```python
from build123d import *

# Parameters (mm, degrees)
F1_DEPTH      = 85
F2_R          = 2.5
F3_DEPTH      = 45
F4_R          = 2.5
F5_DEPTH      = 15
F5_DEPTH_BACK = 25
F6_R          = 1.5
F7_DEPTH      = 15


with BuildPart() as f1:
    # F0 (on Front) → F1 (new body, symmetric)
    with BuildSketch(Plane.XZ):
        Polygon((42, -15), (45, -15), (45, 15), (-45, 15), (-45, -15), (-42, -15), (-42, 12), (42, 12), align=None)
    extrude(amount=F1_DEPTH, both=True)

    # F2 (on Right) → F3 (join, symmetric)
    with BuildSketch(Plane.YZ):
        with Locations((-75, 0)):
            Circle(F2_R)
        with Locations((75, 0)):
            Circle(F2_R)
    extrude(amount=F3_DEPTH, both=True)

    # F4 (on Top) → F5 (join, two sides)
    with BuildSketch(Plane.XY) as f5_sk:
        with Locations((-30, -50)):
            Circle(F4_R)
        with Locations((30, -50)):
            Circle(F4_R)
        with Locations((30, 50)):
            Circle(F4_R)
        with Locations((-30, 50)):
            Circle(F4_R)
    extrude(amount=F5_DEPTH)
    extrude(f5_sk.sketch, amount=-F5_DEPTH_BACK)

    # F6 (on Top) → F7 (cut)
    with BuildSketch(Plane.XY):
        with Locations((-10, 35)):
            Circle(F6_R)
        with Locations((10, 35)):
            Circle(F6_R)
        with Locations((10, -35)):
            Circle(F6_R)
        with Locations((-10, -35)):
            Circle(F6_R)
        with Locations((-15, 35)):
            Circle(F6_R)
        with Locations((15, 35)):
            Circle(F6_R)
        with Locations((15, -35)):
            Circle(F6_R)
        with Locations((-15, -35)):
            Circle(F6_R)
    extrude(amount=F7_DEPTH, mode=Mode.SUBTRACT)


solid = f1.part
```
Model file for the job. Use its own axes, mm. Coordinates: 2 decimals unless noted, no trailing zeros. Loops run counter-clockwise (first coordinate to the right, second up) from the corner with the lowest first, then second, coordinate; pieces in that order, holes last. Notation, with made-up numbers: (40.25, 51) - (53.25, 51) arc R27 ccw to (53.25, 75) - close; hole circle Ø2 at (-14, 11.25). An arc over 180 degrees is marked (long way). Answer as a JSON object with one key per item and string values. Group by question number.
(1) Probe line 1 along Y through (x, z) = (-10, 14); line 2 along X through (y, z) = (35, 12.9); line 3 along X through (y, z) = (-9, -13.5). List the from-to ranges inside material, lowest first.
(2) Cut at B-B (x = 39). Give the cut face in (y, z).
(3) Two-plate mould, pull along X, no slides. Class faces 1 (the face through (-45, -1, 0)), 2 (the face through (0.6, 72.5, 0.1)), 3 (the face through (43, -1, -15)): released by +X, released by -X, zero draft, split by the parting line, or undercut.
(4) Cut at C-C (y = 14). Give the cut face in (x, z), then the cut area to 3 significant figures.
(5) Flat gauge pins, fed straight in: pin 1 (2.5 mm diameter, centred on x = 10, y = 35, fed in from -Z); pin 2 (25 mm diameter, centred on x = 13, y = 35, fed in from -Z); pin 3 (2.5 mm diameter, centred on x = -43.5, y = -5, fed in from -Z). Where does each tip first touch, or does it go through?
(6) Cut at D-D (z = -20.5). Give the cut face in (x, y), then the cut area to 3 significant figures.
(7) Cut at A-A (y = 75). Give the cut face in (x, z), then the cut area to 3 significant figures.
Geometry says:
{
 "1": {"line 1": "y = -85 to -36.5, -33.5 to 33.5, 36.5 to 85", "line 2": "x = -45 to -16.5, -13.5 to -11.5, -8.5 to 8.5, 11.5 to 13.5, 16.5 to 45", "line 3": "x = -45 to -42, 42 to 45"},
 "2": {"outline": "(-85, 12) - (85, 12) - (85, 15) - (-85, 15) - close; circle Ø5 at (-75, 0); circle Ø5 at (75, 0)"},
 "3": {"face 1": "released by -X", "face 2": "undercut", "face 3": "zero draft"},
 "4": {"outline": "(-45, -15) - (-42, -15) - (-42, 12) - (42, 12) - (42, -15) - (45, -15) - (45, 15) - (-45, 15) - close", "area": "432 mm^2"},
 "5": {"pin 1": "passes through", "pin 2": "stops at z = 12", "pin 3": "stops at z = -15"},
 "6": {"outline": "circle Ø5 at (-30, -50); circle Ø5 at (-30, 50); circle Ø5 at (30, -50); circle Ø5 at (30, 50)", "area": "78.5 mm^2"},
 "7": {"outline": "(-45, -15) - (-42, -15) - (-42, -2.5) - (42, -2.5) - (42, -15) - (45, -15) - (45, 15) - (-45, 15) - close; hole (-42, 2.5) - (42, 2.5) - (42, 12) - (-42, 12) - close", "area": "852 mm^2"}
}
